Geometry check sheet. Reference: the model listing, model coordinates, mm. A direction names the side the tool comes from. Give positions to 0.01 mm unless a question says otherwise; leave off trailing zeros. Loops run counter-clockwise (first coordinate to the right, second up) from the corner with the lowest first, then second, coordinate; pieces in that order, holes last.
```python
from build123d import *

# Parameters (mm, degrees)
ESQUISSE1_W             = 330
ESQUISSE1_H             = 54
BOSS_EXTRU_1_DEPTH      = 6
ESQUISSE2_W             = 6
ESQUISSE2_H             = 14
ESQUISSE2_W_2           = 110
ESQUISSE2_H_2           = 6
ENL_V_MAT_EXTRU_1_DEPTH = 335.442820225
ESQUISSE3_R             = 1.5
ESQUISSE3_W             = 6
ESQUISSE3_H             = 20
ENL_V_MAT_EXTRU_2_DEPTH = 6
ESQUISSE4_R             = 2.995
ENL_V_MAT_EXTRU_3_DEPTH = 3


with BuildPart() as part:
    # Esquisse1 → Boss.-Extru.1 (new body)
    with BuildSketch(Plane.XY):
        with Locations((-165, 27)):
            Rectangle(ESQUISSE1_W, ESQUISSE1_H)
    extrude(amount=BOSS_EXTRU_1_DEPTH)

    # Esquisse2 → Enlèv. mat.-Extru.1 (cut, through all)
    with BuildSketch(Plane.XY.offset(6)):
        Polygon((-330, 0), (-240, 0), (-240, 6), (-324, 6), (-324, 20), (-330, 20), align=None)
        Polygon((-90, 6), (-90, 0), (0, 0), (0, 20), (-6, 20), (-6, 6), align=None)
        with Locations((-327, 47)):
            Rectangle(ESQUISSE2_W, ESQUISSE2_H)
        with Locations((-3, 47)):
            Rectangle(ESQUISSE2_W, ESQUISSE2_H)
        with Locations((-165, 3)):
            Rectangle(ESQUISSE2_W_2, ESQUISSE2_H_2)
    extrude(amount=-ENL_V_MAT_EXTRU_1_DEPTH, mode=Mode.SUBTRACT)

    # Esquisse3 → Enlèv. mat.-Extru.2 (cut)
    with BuildSketch(Plane.XY.offset(6)):
        with Locations((-230, 51)):
            Circle(ESQUISSE3_R)
        with Locations((-100, 51)):
            Circle(ESQUISSE3_R)
        with Locations((-3, 30)):
            Rectangle(ESQUISSE3_W, ESQUISSE3_H)
    extrude(amount=-ENL_V_MAT_EXTRU_2_DEPTH, mode=Mode.SUBTRACT)

    # Esquisse4 → Enlèv. mat.-Extru.3 (cut)
    with BuildSketch(Plane.XY.offset(6)):
        with Locations((-230, 51)):
            Circle(ESQUISSE4_R)
        with Locations((-100, 51)):
            Circle(ESQUISSE4_R)
    extrude(amount=-ENL_V_MAT_EXTRU_3_DEPTH, mode=Mode.SUBTRACT)


solid = part.part
```
1) Sectioned sample at C-C on x = -264. Enter the section's corners in (y, z), plus the area to 3 significant figures.
2) Tool access check on faces 5 (the flat face through (-324, 47, 3)), 6 (the flat face through (-90, 3, 3)), 7 (the flat face through (-240, 3, 3)), 8 (the flat face through (-228.7, 49.7, 3)), 9 (the flat face through (-220, 3, 3)). Record the directions out of +Z, -Z, +X, -X, +Y, -Y that give a thin tool (end or side, any length) a straight path to the whole face; none if there is none.
3) Scan lines: line 1 along Y through (x, z) = (-100, 1.8); line 2 along Y through (x, z) = (-83.5, 2); line 3 along X through (y, z) = (40.5, 2.1). Record each from-to range of solid material in increasing order.
4) Mould release check, pull along Y, two halves, no side actions. Record for faces 1 (the flat face through (-110, 3, 3)), 2 (the flat face through (-166, 6, 3)), 3 (the cylindrical face through (-97.143, 51.9, 4.521)), 4 (the flat face through (-98.7, 49.7, 3)): +Y half, -Y half, draft (parallel to the pull), parting line (faces both ways), or undercut.
5) Sectioned sample at B-B on y = 14.5. Enter the section's corners in (x, z), plus the area to 3 significant figures.
6) Sectioned sample at A-A on z = 4.5. Enter the section's corners in (x, y) (3 decimals), plus the area to 3 significant figures.
7) Depth check by flat-ended pin: P1, Ø3, axis at y = 4, z = 2.5, coming from the -X side; P2, Ø1.8, axis at y = 2, z = 3, coming from the +X side; P3, Ø2.5, axis at x = -230, y = 51, coming from the +Z side; P4, Ø2, axis at y = 18, z = 1.5, coming from the -X side. Enter the tip coordinate at first touch or a pass-through.
Determined:
1. outline: (6, 0) - (54, 0) - (54, 6) - (6, 6) - close
1. area: 288 mm2
2. face 5: +Z, -Z, -X, +Y
2. face 6: +Z, -Z, +X, -Y
2. face 7: +Z, -Z, -X, -Y
2. face 8: +Z
2. face 9: +Z, -Z, -Y
3. line 1: y = 0 to 49.5, 52.5 to 54
3. line 2: y = 6 to 54
3. line 3: x = -324 to -6
4. face 1: draft
4. face 2: -Y half
4. face 3: undercut
4. face 4: undercut
5. outline: (-324, 0) - (-6, 0) - (-6, 6) - (-324, 6) - close
5. area: 1,910 mm2
6. outline: (-330, 20) - (-324, 20) - (-324, 6) - (-240, 6) - (-240, 0) - (-220, 0) - (-220, 6) - (-110, 6) - (-110, 0) - (-90, 0) - (-90, 6) - (-6, 6) - (-6, 54) - (-324, 54) - (-324, 40) - (-330, 40) - close; hole circle Ø5.99 at (-230, 51); hole circle Ø5.99 at (-100, 51)
6. area: 15,600 mm2
7. P1: stops at x = -240
7. P2: stops at x = -90
7. P3: passes through
7. P4: stops at x = -324
